```python
from build123d import *

# Parameters (mm, degrees)
F1_DEPTH = 3
F2_R     = 1.5
F3_W     = 3.302
F3_H     = 1.6
F3_W_2   = 1.6
F3_H_2   = 3.302
F4_DEPTH = 3.001


with BuildPart() as f1:
    # F0 (on Top) → F1 (new body)
    with BuildSketch(Plane.XY):
        Polygon((-30.010116, 45), (-30.010116, 0), (47.93217, 0), align=None)
        Polygon((29.271916, 5), (-25.010116, 5), (-25.010116, 36.339746), align=None, mode=Mode.SUBTRACT)
    extrude(amount=F1_DEPTH)

    # F2
    f2_edges = [f1.edges().sort_by_distance(p)[0] for p in [
        (-25.010116, 36.339746, 1.5),
        (29.271916, 5, 1.5),
        (-25.010116, 5, 1.5),
    ]]
    fillet(f2_edges, radius=F2_R)

    # F3 (on face) → F4 (cut, through all)
    with BuildSketch(Plane.XY.offset(3)):
        Polygon((-28.410116, 35.125), (-28.410116, 33.651), (-28.410116, 30.349), (-28.410116, 28.875), (-26.110116, 28.875), (-26.110116, 35.125), align=None)
        Polygon((-28.410116, 13.651), (-28.410116, 10.349), (-28.410116, 8.875), (-26.110116, 8.875), (-26.110116, 15.125), (-28.410116, 15.125), align=None)
        Polygon((-19.661116, 1.6), (-16.359116, 1.6), (-14.885116, 1.6), (-14.885116, 3.9), (-21.135116, 3.9), (-21.135116, 1.6), align=None)
        Polygon((21.640884, 1.6), (23.114884, 1.6), (23.114884, 3.9), (16.864884, 3.9), (16.864884, 1.6), (18.338884, 1.6), align=None)
        with Locations((19.989884, 0.8)):
            Rectangle(F3_W, F3_H)
        with Locations((-29.210116, 32)):
            Rectangle(F3_W_2, F3_H_2)
        with Locations((-18.010116, 0.8)):
            Rectangle(F3_W, F3_H)
        with Locations((-29.210116, 12)):
            Rectangle(F3_W_2, F3_H_2)
    extrude(amount=-F4_DEPTH, mode=Mode.SUBTRACT)


solid = f1.part
```
Input: part model. Units: mm. Frame: model coordinates. A direction names the side the tool comes from. Round coordinates to 2 decimals unless told otherwise and drop trailing zeros. Loops run counter-clockwise (first coordinate to the right, second up) from the corner with the lowest first, then second, coordinate; pieces in that order, holes last. Notation, with made-up numbers: (12.5, 19) -> (25.5, 19) arc R19 ccw to (25.5, 33) -> close; hole circle Ø7 at (66, 0.5). An arc over 180 degrees is marked (long way). Write each question's results on one line, items separated by ' | '.
1. Section C-C (x = 31.5). Return loops of the section in (y, z).
Geometry results:
outline: (0, 0) -> (9.49, 0) -> (9.49, 3) -> (0, 3) -> close
2. Set-up query: faces 1 (the face through (23.115, 3, 2)), 2 (the face through (-16.359, 1, 2)), 3 (the face through (-29, 33.651, 2)). Return all of +Z, -Z, +X, -X, +Y, -Y with unobstructed straight access to the full face (end or side cutting, diameter ignored); none if empty.
Geometry results:
face 1: +Z, -Z | face 2: +Z, -Z, -Y | face 3: +Z, -Z, -X
3. Section B-B (y = 23). Return loops of the section in (x, z) (3 decimals), and give its area (3 significant figures).
Geometry results:
outline: (-30.01, 0) -> (-25.01, 0) -> (-25.01, 3) -> (-30.01, 3) -> close; (-1.905, 0) -> (8.095, 0) -> (8.095, 3) -> (-1.905, 3) -> close | area: 45.0 mm2
4. First-contact query: P1, Ø1, axis at y = 31.5, z = 2, coming from the +X side; P2, Ø0.9, axis at y = 31.5, z = 2, coming from the -X side; P3, Ø1.5, axis at x = 8, z = 1.5, coming from the +Y side. Flat tips, straight axial feed; report the tip coordinate or a pass-through.
Geometry results:
P1: x = -5.76 | P2: x = -26.11 | P3: y = 23.49
5. Ray query, line 1 (X direction, y = 9, z = 2.5); line 2 (Y direction, x = 22, z = 1); line 3 (X direction, y = 9.5, z = 0.65). Return the intervals inside material, ascending. Write a range as from..to.
Geometry results:
line 1: -30.01..-28.41, -26.11..-25.01, 22.34..32.34 | line 2: 0..1.6, 3.9..5, 9.2..14.97 | line 3: -30.01..-28.41, -26.11..-25.01, 21.48..31.48
6. Section A-A (x = 14). Return loops of the section in (y, z).
Geometry results:
outline: (0, 0) -> (5, 0) -> (5, 3) -> (0, 3) -> close; (13.82, 0) -> (19.59, 0) -> (19.59, 3) -> (13.82, 3) -> close
7. Mould query, pull axis X, two halves, no side actions, for faces 4 (the face through (16.865, 3, 2)), 5 (the face through (-30.01, 5, 1)), 6 (the face through (-29, 30.349, 2)). Classes: +X half, -X half, draft (parallel to the pull), parting line (faces both ways), or undercut.
Geometry results:
face 4: undercut | face 5: -X half | face 6: draft
